Autodesk Inventor part; units mm, degrees
ref_plane "YZ Plane" through (0, 0, 0) normal (1, 0, 0) x (0, 1, 0)
ref_plane "XZ Plane" through (0, 0, 0) normal (0, 1, 0) x (-1, 0, 0)
ref_plane "XY Plane" through (0, 0, 0) normal (0, 0, 1) x (1, 0, 0)
sketch "Sketch1" plane through (0, 0, 0) normal (0, 1, 0) x (-1, 0, 0)
  line L0 (0, -170) -> (260, -170)
  line L1 (260, -170) -> (260, 0)
  line L2 (260, 0) -> (0, 0)
  line L3 (0, 0) -> (0, -170)
  dimension "d2" = 260
  dimension "d3" = 170
extrude "Box" add sketch "Sketch1" along normal blind 50
sketch "Sketch2" plane through (0, 0, 0) normal (1, 0, 0) x (0, 0, -1)
  line L0 (35, 14) -> (21, 14)
  line L1 (20, 15) -> (20, 28.2)
  line L2 (21, 29.2) -> (35, 29.2)
  line L3 (36, 28.2) -> (36, 15)
  arc A0 (21, 29.2) -> (20, 28.2) centre (21, 28.2) ccw
  arc A1 (36, 28.2) -> (35, 29.2) centre (35, 28.2) ccw
  arc A2 (35, 14) -> (36, 15) centre (35, 15) ccw
  arc A3 (20, 15) -> (21, 14) centre (21, 15) ccw
  line L4 (65, 14) -> (51, 14)
  line L5 (50, 15) -> (50, 28.2)
  line L6 (51, 29.2) -> (65, 29.2)
  line L7 (66, 28.2) -> (66, 15)
  arc A4 (51, 29.2) -> (50, 28.2) centre (51, 28.2) ccw
  arc A5 (66, 28.2) -> (65, 29.2) centre (65, 28.2) ccw
  arc A6 (65, 14) -> (66, 15) centre (65, 15) ccw
  arc A7 (50, 15) -> (51, 14) centre (51, 15) ccw
  line L8 (95, 14) -> (81, 14)
  line L9 (80, 15) -> (80, 28.2)
  line L10 (81, 29.2) -> (95, 29.2)
  line L11 (96, 28.2) -> (96, 15)
  arc A8 (81, 29.2) -> (80, 28.2) centre (81, 28.2) ccw
  arc A9 (96, 28.2) -> (95, 29.2) centre (95, 28.2) ccw
  arc A10 (95, 14) -> (96, 15) centre (95, 15) ccw
  arc A11 (80, 15) -> (81, 14) centre (81, 15) ccw
  line L12 (125, 14) -> (111, 14)
  line L13 (110, 15) -> (110, 28.2)
  line L14 (111, 29.2) -> (125, 29.2)
  line L15 (126, 28.2) -> (126, 15)
  arc A12 (111, 29.2) -> (110, 28.2) centre (111, 28.2) ccw
  arc A13 (126, 28.2) -> (125, 29.2) centre (125, 28.2) ccw
  arc A14 (125, 14) -> (126, 15) centre (125, 15) ccw
  arc A15 (110, 15) -> (111, 14) centre (111, 15) ccw
  line L16 (0, 0) -> (0, 50) construction
  line L17 (0, 0) -> (170, 0) construction
  point P0 (36, 14)
  point P1 (20, 29.2)
  point P2 (20, 14)
  point P3 (36, 29.2)
  point P4 (66, 14)
  point P5 (50, 29.2)
  point P6 (50, 14)
  point P7 (66, 29.2)
  point P8 (96, 14)
  point P9 (80, 29.2)
  point P10 (80, 14)
  point P11 (96, 29.2)
  point P12 (126, 14)
  point P13 (110, 29.2)
  point P14 (110, 14)
  point P15 (126, 29.2)
  point P16 (20, 21.6)
  point P17 (28, 29.2)
  dimension "d6" = 16
  dimension "d72" = 1
  dimension "d73" = 16
  dimension "d75" = 1
  dimension "d76" = 16
  dimension "d78" = 1
  dimension "d79" = 16
  dimension "d81" = 1
  dimension "d82" = 14
  dimension "d83" = 20
  dimension "d84" = 30
  dimension "d87" = 30
  dimension "d88" = 30
  dimension "d110" = 15.2
extrude "Ethernet" cut sketch "Sketch2" against normal blind 20
sketch "Sketch6" plane through (-260, 0, 0) normal (0, 0, 1) x (1, 0, 0)
  line L0 (40, 29.2) -> (26, 29.2)
  line L1 (25, 28.2) -> (25, 15)
  line L2 (26, 14) -> (40, 14)
  line L3 (41, 15) -> (41, 28.2)
  line L4 (0, 0) -> (0, 50)
  line L5 (0, 0) -> (260, 0)
  arc A0 (26, 29.2) -> (25, 28.2) centre (26, 28.2) ccw
  arc A1 (41, 28.2) -> (40, 29.2) centre (40, 28.2) ccw
  arc A2 (40, 14) -> (41, 15) centre (40, 15) ccw
  arc A3 (25, 15) -> (26, 14) centre (26, 15) ccw
  line L6 (69, 29.2) -> (55, 29.2)
  line L7 (54, 28.2) -> (54, 15)
  line L8 (55, 14) -> (69, 14)
  line L9 (70, 15) -> (70, 28.2)
  arc A4 (55, 29.2) -> (54, 28.2) centre (55, 28.2) ccw
  arc A5 (70, 28.2) -> (69, 29.2) centre (69, 28.2) ccw
  arc A6 (69, 14) -> (70, 15) centre (69, 15) ccw
  arc A7 (54, 15) -> (55, 14) centre (55, 15) ccw
  point P0 (41, 29.2)
  point P1 (25, 14)
  point P2 (25, 29.2)
  point P3 (41, 14)
  point P4 (70, 29.2)
  point P5 (54, 14)
  point P6 (54, 29.2)
  point P7 (70, 14)
  dimension "d22" = 16
  dimension "d23" = 15.2
  dimension "d92" = 25
  dimension "d93" = 14
  dimension "d94" = 1
  dimension "d95" = 16
  dimension "d97" = 1
  dimension "d99" = 13
extrude "Rotary-Ethernet" cut sketch "Sketch6" against normal blind 20
sketch "Sketch9" plane through (0, 50, 0) normal (0, 1, 0) x (1, 0, 0)
  circle A0 centre (-235, 120) radius 2.5
  line L0 (-260, 170) -> (-260, 0) construction
  line L1 (0, 170) -> (-260, 170) construction
  circle A1 centre (-235, 145) radius 2.5
  point P0 (0, 0)
  dimension "d33" = 5
  dimension "d68" = 25
  dimension "d69" = 50
  dimension "d70" = 25
  dimension "d71" = 25
extrude "Spout1" cut sketch "Sketch9" against normal blind 20
sketch "Sketch11" plane through (0, 0, -170) normal (0, 0, -1) x (-1, 0, 0)
  line L0 (146, 14) -> (126, 14)
  line L1 (125, 15) -> (125, 28)
  line L2 (126, 29) -> (146, 29)
  line L3 (147, 28) -> (147, 15)
  line L4 (0, 0) -> (260, 0)
  line L5 (0, 0) -> (0, 50)
  arc A0 (126, 29) -> (125, 28) centre (126, 28) ccw
  arc A1 (147, 28) -> (146, 29) centre (146, 28) ccw
  arc A2 (146, 14) -> (147, 15) centre (146, 15) ccw
  arc A3 (125, 15) -> (126, 14) centre (126, 15) ccw
  point P0 (0, 0)
  point P1 (147, 14)
  point P2 (125, 29)
  point P3 (125, 14)
  point P4 (147, 29)
  dimension "d39" = 22
  dimension "d40" = 15
  dimension "d105" = 14
  dimension "d106" = 125
  dimension "d107" = 1
extrude "Teensy usb" cut sketch "Sketch11" against normal blind 10
sketch "Sketch13" plane through (-260, 0, 0) normal (0, 0, 1) x (1, 0, 0)
  line L0 (220, 29.2) -> (234, 29.2)
  line L1 (235, 28.2) -> (235, 15)
  line L2 (234, 14) -> (220, 14)
  line L3 (219, 15) -> (219, 28.2)
  line L4 (260, 0) -> (260, 50)
  line L5 (0, 0) -> (260, 0)
  arc A0 (220, 29.2) -> (219, 28.2) centre (220, 28.2) ccw
  arc A1 (235, 28.2) -> (234, 29.2) centre (234, 28.2) ccw
  arc A2 (234, 14) -> (235, 15) centre (234, 15) ccw
  arc A3 (219, 15) -> (220, 14) centre (220, 15) ccw
  point P0 (219, 29.2)
  point P1 (235, 14)
  point P2 (235, 29.2)
  point P3 (219, 14)
  dimension "d43" = 16
  dimension "d44" = 15.2
  dimension "d89" = 25
  dimension "d90" = 14
  dimension "d91" = 1
extrude "Teensy shield" cut sketch "Sketch13" against normal blind 10
sketch "power 5 v" plane through (0, 0, -170) normal (0, 0, -1) x (-1, 0, 0)
  circle A0 centre (122, 14) radius 6.5
  line L0 (0, 0) -> (260, 0)
  line L1 (146, 14) -> (126, 14)
  point P0 (136, 14)
  dimension "d47" = 13
  dimension "d108" = 14
  dimension "d109" = 14
extrude "Power5" cut sketch "power 5 v" against normal blind 20
sketch "power9" plane through (0, 0, 0) normal (1, 0, 0) x (0, 0, -1)
  circle A0 centre (145, 14) radius 6.5
  line L0 (0, 0) -> (170, 0)
  line L1 (170, 0) -> (170, 50)
  dimension "d50" = 13
  dimension "d85" = 14
  dimension "d86" = 25
extrude "Power 9" cut sketch "power9" against normal blind 20
sketch "Power121" plane through (-260, 0, 0) normal (0, 0, 1) x (1, 0, 0)
  circle A0 centre (175, 14) radius 6.5
  line L0 (0, 0) -> (260, 0)
  arc A1 (234, 14) -> (235, 15) centre (234, 15) ccw
  line L1 (234, 14) -> (220, 14)
  arc A2 (219, 15) -> (220, 14) centre (220, 15) ccw
  line L2 (219, 15) -> (219, 28.2)
  arc A3 (220, 29.2) -> (219, 28.2) centre (220, 28.2) ccw
  line L3 (220, 29.2) -> (234, 29.2)
  arc A4 (235, 28.2) -> (234, 29.2) centre (234, 28.2) ccw
  line L4 (235, 28.2) -> (235, 15)
  line L5 (25, 15) -> (25, 28.2)
  arc A5 (26, 29.2) -> (25, 28.2) centre (26, 28.2) ccw
  line L6 (26, 29.2) -> (40, 29.2)
  arc A6 (41, 28.2) -> (40, 29.2) centre (40, 28.2) ccw
  line L7 (41, 28.2) -> (41, 15)
  arc A7 (40, 14) -> (41, 15) centre (40, 15) ccw
  line L8 (40, 14) -> (26, 14)
  arc A8 (25, 15) -> (26, 14) centre (26, 15) ccw
  arc A9 (55, 29.2) -> (54, 28.2) centre (55, 28.2) ccw
  line L9 (55, 29.2) -> (69, 29.2)
  arc A10 (70, 28.2) -> (69, 29.2) centre (69, 28.2) ccw
  line L10 (70, 28.2) -> (70, 15)
  arc A11 (69, 14) -> (70, 15) centre (69, 15) ccw
  line L11 (69, 14) -> (55, 14)
  arc A12 (54, 15) -> (55, 14) centre (55, 15) ccw
  line L12 (54, 15) -> (54, 28.2)
  line L13 (0, 0) -> (260, 0)
  line L14 (260, 0) -> (260, 50)
  line L15 (0, 50) -> (260, 50)
  line L16 (0, 0) -> (0, 50)
  dimension "d53" = 13
  dimension "d100" = 14
  dimension "d101" = 85
extrude "Power12" cut sketch "Power121" against normal blind 20 contours A0
sketch "Rotary USB1" plane through (-260, 0, -170) normal (-1, 0, 0) x (0, 0, 1)
  line L0 (137, 29) -> (117, 29)
  line L1 (116, 28) -> (116, 15)
  line L2 (117, 14) -> (137, 14)
  line L3 (138, 15) -> (138, 28)
  line L4 (0, 0) -> (170, 0)
  line L5 (170, 0) -> (170, 50)
  arc A0 (138, 28) -> (137, 29) centre (137, 28) ccw
  arc A1 (137, 14) -> (138, 15) centre (137, 15) ccw
  arc A2 (116, 15) -> (117, 14) centre (117, 15) ccw
  arc A3 (117, 29) -> (116, 28) centre (117, 28) ccw
  point P0 (170, 0)
  point P1 (138, 29)
  point P2 (116, 14)
  point P3 (116, 29)
  point P4 (138, 14)
  dimension "d58" = 22
  dimension "d59" = 15
  dimension "d102" = 14
  dimension "d103" = 32
  dimension "d104" = 1
extrude "Rotary USB" cut sketch "Rotary USB1" against normal blind 20
sketch "Sketch19" plane through (0, 0, 0) normal (0, -1, 0) x (1, 0, 0)
  line L0 (-260, -170) -> (-260, 0) construction
  line L1 (0, -170) -> (-260, -170) construction
  line L2 (0, 0) -> (0, -170) construction
  line L3 (-260, 0) -> (0, 0) construction
  line L4 (-8, -162) -> (-252, -162)
  line L5 (-252, -162) -> (-252, -8)
  line L6 (-252, -8) -> (-8, -8)
  line L7 (-8, -8) -> (-8, -162)
  dimension "d62" = 8
  dimension "d63" = 8
  dimension "d64" = 8
  dimension "d65" = 8
extrude "Extrusion17" cut sketch "Sketch19" against normal blind 46
fillet "Fillet1" radius 2 2 edges at (-128.5, 14, -166) (-125, 19.7663, -166)
sketch "Sketch20" plane through (-260, 0, -170) normal (-1, 0, 0) x (0, 0, 1)
  circle A0 centre (90, 24) radius 12.5
  line L0 (0, 0) -> (170, 0)
  line L1 (0, 0) -> (0, 50)
  dimension "d112" = 25
  dimension "d113" = 24
  dimension "d114" = 90
extrude "Extrusion18" cut sketch "Sketch20" against normal blind 20
properties part number "TouchShakerBox"
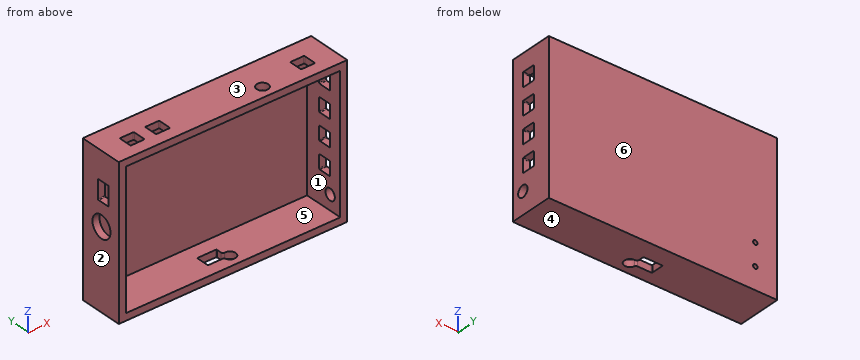
The model under review builds one solid part; all positions refer to its coordinate system, in mm. Face numbers are marked on the shaded views. A direction names the side the tool comes from. Give positions to 0.01 mm unless a question says otherwise; leave off trailing zeros. Write each loop counter-clockwise with the first axis right and the second up, starting at its lowest first coordinate (ties: lowest second). Pieces come first, ordered by that corner, then holes. Notation, with made-up numbers: M 81,72 L 89,72 A7 cw 89,81 Z; hole C -14,63 d11. An arc over 180 degrees is marked long. Write item = value, one per line. Start each with the question number.
Q1. We need section B-B (z = -71.5). State the section outline as (x, y) points, plus the area to 3 significant figures.
Q2. Machinability: for the marked faces 5 and 6, which of the approach directions +Z, -Z, +X, -X, +Y, -Y give a long, thin tool a straight path to every point of the face, cutting with its end or side? Answer none if there is none.
Q3. We need section D-D (x = -242). State the section outline as (y, z) points.
Q4. We need section C-C (z = -158.5). State the section outline as (x, y) points.
Q5. Mouldability with a two-part tool opening along Z and no side actions: class the marked faces 1, 2, 3 and 4 as released by +Z, released by -Z, zero draft, split by the parting line, or undercut.
Q6. We need section A-A (x = -87.5). State the section outline as (y, z) points.
Q7. Clearance check with flat-ended pins moving along their axes: pin 1 (6 mm diameter, centred on x = -99, z = -66.5, fed in from -Y); pin 2 (2.5 mm diameter, centred on x = -36, z = -5, fed in from -Y); pin 3 (8 mm diameter, centred on y = 14, z = -145, fed in from +X). State where each tip first meets the part, or that it passes through.
Q8. For line 1 (Z direction, x = -29, y = 7.5); line 2 (X direction, y = 22.5, z = -135.5); line 3 (X direction, y = 47.8, z = -145), list the stretches that pass through material, from the lowest coordinate up.
Result set:
q1.outline = M -260,0 L -252,0 L -252,14.83 L -260,14.83 Z; M -260,33.17 L -252,33.17 L -252,46 L -8,46 L -8,0 L 0,0 L 0,50 L -260,50 Z
q1.area = 1,630 mm2
q2.face_5 = -Y
q2.face_6 = +Z, -Z, +X, -X, +Y
q3.outline = M 0,-170 L 50,-170 L 50,0 L 0,0 L 0,-8 L 46,-8 L 46,-162 L 0,-162 Z
q4.outline = M -260,0 L -252,0 L -252,46 L -8,46 L -8,0 L 0,0 L 0,50 L -260,50 Z
q5.face_1 = undercut
q5.face_2 = zero draft
q5.face_3 = released by +Z
q5.face_4 = released by -Z
q6.outline = M 0,-170 L 50,-170 L 50,0 L 20,0 L 20,-8 L 46,-8 L 46,-162 L 0,-162 Z; M 0,-8 L 8,-8 L 8,0 L 0,0 Z
q7.pin_1 = 46
q7.pin_2 = 0
q7.pin_3 = -252
q8.line_1 = -170 to -162, -8 to 0
q8.line_2 = -260 to -252, -8 to 0
q8.line_3 = -260 to -237.5, -232.5 to 0
